Input: dimensioned drawing with shaded views. Units: mm. Origin: part minimum x, y, z. A direction names the side the tool comes from. Give positions to 0.01 mm unless a question says otherwise; leave off trailing zeros. Order: outer loops, then holes, each group sorted by start corner. A loop starts at its lowest first (then second) coordinate and runs counter-clockwise, first axis right, second up. Notation, with made-up numbers: M 60,86 L 68,86 A23 ccw 68,112 Z; hole C 84.5,43 d3. An arc over 180 degrees is marked long. Answer in a Markdown table with one row per item. Add a question column.
(1) Section query C-C, the plane x = 3.25. Return loops of the section in (y, z).
(2) Material intervals for line 1 along Y through (x, z) = (4.75, 7.5); line 2 along X through (y, z) = (4, 2.75); line 3 along Y through (x, z) = (10.5, 8.5), sorted ascending.
(3) Set-up query: the marked faces 4 and 5. Return all of +Z, -Z, +X, -X, +Y, -Y with unobstructed straight access to the full face (end or side cutting, diameter ignored); none if empty.
(4) Pin query (flat end, axial travel): P1, Ø6, axis at x = 7, y = 4, coming from the +Z side; P2, Ø5, axis at x = 10, y = 13.5, coming from the -Z side; P3, Ø4, axis at x = 12.5, z = 5, coming from the -Y side. Return the tip coordinate at first contact, or that it passes through.
(5) Mould query, pull axis Y, two halves, no side actions, for the marked faces 1, 2 and 3. Classes: pulls with the +Y half, pulls with the -Y half, needs draft (parallel to the pull), parting line crosses it, or undercut.
(6) Section query A-A, the plane z = 7.5. Return loops of the section in (x, y).
(7) Section query D-D, the plane x = 15.5. Return loops of the section in (y, z).
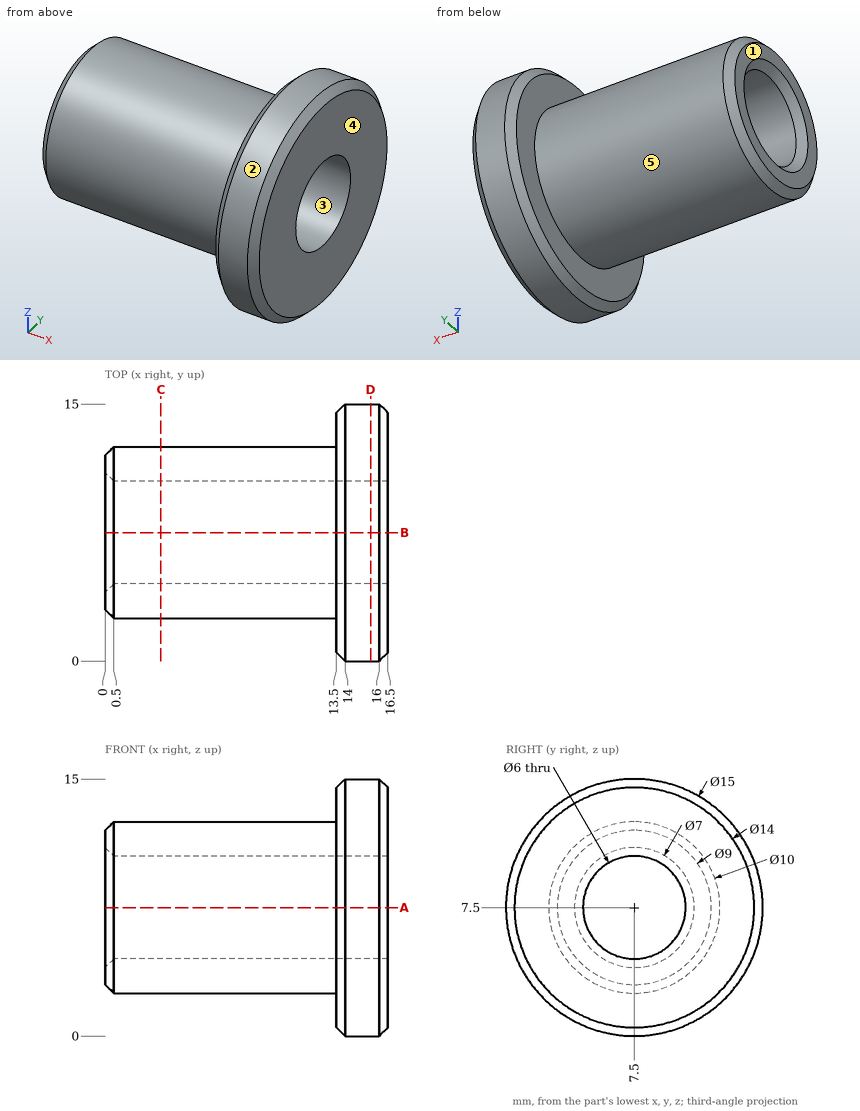
Values follow:
| question | item | result |
|---|---|---|
| 1 | outline | C 7.5,7.5 d10; hole C 7.5,7.5 d6 |
| 2 | line 1 | y = 2.5 to 4.5, 10.5 to 12.5 |
| 2 | line 2 | x = 13.5 to 16.5 |
| 2 | line 3 | y = 2.6 to 4.67, 10.33 to 12.4 |
| 3 | face 4 | +Z, -Z, +X, +Y, -Y |
| 3 | face 5 | -X |
| 4 | P1 | stops at z = 12.47 |
| 4 | P2 | stops at z = 3.93 |
| 4 | P3 | stops at y = 0.09 |
| 5 | face 1 | needs draft |
| 5 | face 2 | parting line crosses it |
| 5 | face 3 | undercut |
| 6 | outline | M 0,3 L 0.5,2.5 L 13.5,2.5 L 13.5,0.5 L 14,0 L 16,0 L 16.5,0.5 L 16.5,4.5 L 0.5,4.5 L 0,4 Z; M 0,11 L 0.5,10.5 L 16.5,10.5 L 16.5,14.5 L 16,15 L 14,15 L 13.5,14.5 L 13.5,12.5 L 0.5,12.5 L 0,12 Z |
| 7 | outline | C 7.5,7.5 d15; hole C 7.5,7.5 d6 |
